from build123d import *

# Parameters (mm, degrees)
SKETCH1_R               = 12.5
SKETCH1_R_2             = 7.5
SKETCH1_R_3             = 12
SKETCH1_R_4             = 9
SKETCH1_W               = 167.634848648
SKETCH1_H               = 10
BOSS_EXTRUDE1_DEPTH     = 58
SKETCH2_W               = 22.908712115
SKETCH2_H               = 11
SKETCH2_W_2             = 18.043560763
SKETCH2_H_2             = 20
SKETCH2_W_3             = 23.956439237
CUT_EXTRUDE1_DEPTH      = 8.5
CUT_EXTRUDE1_DEPTH_BACK = 18.5
BOSS_EXTRUDE2_START     = -0.99133
BOSS_EXTRUDE2_DEPTH     = 0.99133
BOSS_EXTRUDE3_START     = -4.717797
BOSS_EXTRUDE3_DEPTH     = 4.717797
FILLET1_R               = 5
FILLET2_R               = 8
FILLET3_R               = 10


with BuildPart() as part:
    # Sketch1 → Boss-Extrude1 (new body)
    with BuildSketch(Plane(origin=(0, 0, 0), x_dir=(1, 0, 0), z_dir=(0, 1, 0))):
        Circle(SKETCH1_R)
        Circle(SKETCH1_R_2, mode=Mode.SUBTRACT)
        with Locations((190, 0)):
            Circle(SKETCH1_R_3)
        with Locations((190, 0)):
            Circle(SKETCH1_R_4, mode=Mode.SUBTRACT)
        with Locations((95.273863561, 0)):
            Rectangle(SKETCH1_W, SKETCH1_H)
    extrude(amount=BOSS_EXTRUDE1_DEPTH)

    # Sketch2 → Cut-Extrude1 (cut, two sides)
    with BuildSketch(Plane(origin=(0, 0, -5), x_dir=(-1, 0, 0), z_dir=(0, 0, -1))) as cut_extrude1_sk:
        with Locations((-190.545643943, 52.5)):
            Rectangle(SKETCH2_W, SKETCH2_H)
        Polygon((-179.091287885, 47), (-179.091287885, 46.00867027), (-11.456439237, 53.327765826), (-11.456439237, 58), (-179.091287885, 58), align=None)
        with Locations((-190.545643943, 5.5)):
            Rectangle(SKETCH2_W, SKETCH2_H)
        Polygon((-179.091287885, 11.99132973), (-179.091287885, 11), (-179.091287885, 0), (-11.456439237, 0), (-11.456439237, 4.672234174), align=None)
        Polygon((-170.091287885, 19.606002726), (-170.091287885, 38.393997274), (-125.091287885, 40.358739705), (-125.091287885, 17.641260295), align=None)
        Polygon((-115.091287885, 17.204650866), (-115.091287885, 40.795349134), (-40.091287885, 44.069919853), (-40.091287885, 13.930080147), align=None)
        with Locations((-20.478219619, 29)):
            Rectangle(SKETCH2_W_2, SKETCH2_H_2)
        with Locations((0.521780381, 29)):
            Rectangle(SKETCH2_W_3, SKETCH2_H_2)
    extrude(amount=CUT_EXTRUDE1_DEPTH, mode=Mode.SUBTRACT)
    extrude(cut_extrude1_sk.sketch, amount=-CUT_EXTRUDE1_DEPTH_BACK, mode=Mode.SUBTRACT)

    # Sketch3 → Boss-Extrude2 (add)
    with BuildSketch(Plane.XZ.offset(-11).offset(BOSS_EXTRUDE2_START)):
        with BuildLine():
            Line((179.091287885, -5), (179.091287885, 5))
            ThreePointArc((179.091287885, 5), (178, 0), (179.091287885, -5))
        make_face()
    boss_extrude2 = extrude(amount=BOSS_EXTRUDE2_DEPTH)

    # Sketch4 → Boss-Extrude3 (add)
    with BuildSketch(Plane.XZ.offset(BOSS_EXTRUDE3_START)):
        with BuildLine():
            Line((11.456439237, 5), (11.456439237, -5))
            ThreePointArc((11.456439237, -5), (12.236328912, -2.553870546), (12.5, 0))
            ThreePointArc((12.5, 0), (12.236328912, 2.553870546), (11.456439237, 5))
        make_face()
    boss_extrude3 = extrude(amount=BOSS_EXTRUDE3_DEPTH)

    # Mirror1: Boss-Extrude2, Boss-Extrude3 across plane
    add(boss_extrude2.mirror(Plane(origin=(0, 29, 0), x_dir=(0, 0, 1), z_dir=(0, -1, 0))))
    add(boss_extrude3.mirror(Plane(origin=(0, 29, 0), x_dir=(0, 0, 1), z_dir=(0, -1, 0))))

    # Fillet1
    fillet1_edges = [part.edges().sort_by_distance(p)[0] for p in [
        (170.091287885, 19.606002726, 0),
        (170.091287885, 38.393997274, 0),
    ]]
    fillet(fillet1_edges, radius=FILLET1_R)

    # Fillet2
    fillet2_edges = [part.edges().sort_by_distance(p)[0] for p in [
        (115.091287885, 17.204650866, 0),
        (115.091287885, 40.795349134, 0),
        (125.091287885, 40.358739705, 0),
        (125.091287885, 17.641260295, 0),
    ]]
    fillet(fillet2_edges, radius=FILLET2_R)

    # Fillet3
    fillet3_edges = [part.edges().sort_by_distance(p)[0] for p in [
        (40.091287885, 44.069919853, 0),
        (40.091287885, 13.930080147, 0),
    ]]
    fillet(fillet3_edges, radius=FILLET3_R)


solid = part.part
The listing builds one solid part. Answer for the finished solid, in the listing's coordinates (mm). A direction names the side the tool comes from. Give positions to 0.01 mm unless a question says otherwise; leave off trailing zeros. Write each loop counter-clockwise with the first axis right and the second up, starting at its lowest first coordinate (ties: lowest second). Pieces come first, ordered by that corner, then holes. Notation, with made-up numbers: (30.5, -12) - (58.5, -12) arc R21 cw to (58.5, 24) - close; hole circle Ø10 at (23, 70.25). An arc over 180 degrees is marked (long way). One line per question, with ' | ' between items. Start each with the question number.
1. Section A-A, the plane x = 190 is taken. Determine the outline of the cut face in (y, z).
2. Section C-C, the plane x = 81.5 is taken. Determine the outline of the cut face in (y, z), then the cut area to 3 significant figures.
3. Straight lines are drawn through the part: line 1 (X direction, y = 54, z = -0.75); line 2 (X direction, y = 13, z = -5.25); line 3 (Z direction, x = 0, y = 14.75). For each, find the intervals that lie inside material, in ascending order.
4. For faces 1 (the face through (8, 39, 0)), 2 (the face through (168.74, 20.974, 0.07)), 3 (the face through (75, 45, -5)), 4 (the face through (192, 11, 9)), 5 (the face through (0, 58, -8)), determine the directions among +Z, -Z, +X, -X, +Y, -Y from which every point of the face is accessible in a straight line to the end or side of a thin tool.
5. Given P1, Ø10, axis at x = 140.5, y = 46.5, coming from the +Z side; P2, Ø7.5, axis at x = 17.5, z = -0.5, coming from the +Y side; P3, Ø1.5, axis at x = 17.5, y = 48.5, coming from the -Z side, each flat-ended and moving along its own axis, determine where each tip first touches the part or whether it passes through.
6. Section B-B, the plane x = 0 is taken. Determine the outline of the cut face in (y, z).
7. Determine the mould class of faces 6 (the face through (149.15, 18.69, -0.07)), 7 (the face through (9, 19, 0)) for opening direction X: +X half, -X half, draft (parallel to the pull), parting line (faces both ways), or undercut.
Result:
1) outline: (11, -12) - (47, -12) - (47, -9) - (11, -9) - close; (11, 9) - (47, 9) - (47, 12) - (11, 12) - close
2) outline: (7.73, -5) - (15.74, -5) - (15.74, 5) - (7.73, 5) - close; (42.26, -5) - (50.27, -5) - (50.27, 5) - (42.26, 5) - close | area: 160 mm2
3) line 1: x = -12.48 to -7.46, 7.46 to 12.48 | line 2: x = -11.34 to -5.36, 5.36 to 11.34, 179.21 to 182.69, 197.31 to 200.79 | line 3: z = -12.5 to -7.5, 7.5 to 12.5
4) face 1: +Z, -Z, -X | face 2: +Z, -Z | face 3: -Z, +Y, -Y | face 4: +Z, -Z, +X, -Y | face 5: +Z, -Z, +X, -X, +Y
5) P1: stops at z = 5 | P2: stops at y = 53.23 | P3: stops at z = -5
6) outline: (0, -12.5) - (19, -12.5) - (19, -7.5) - (0, -7.5) - close; (0, 7.5) - (19, 7.5) - (19, 12.5) - (0, 12.5) - close; (39, -12.5) - (58, -12.5) - (58, -7.5) - (39, -7.5) - close; (39, 7.5) - (58, 7.5) - (58, 12.5) - (39, 12.5) - close
7) face 6: undercut | face 7: draft
